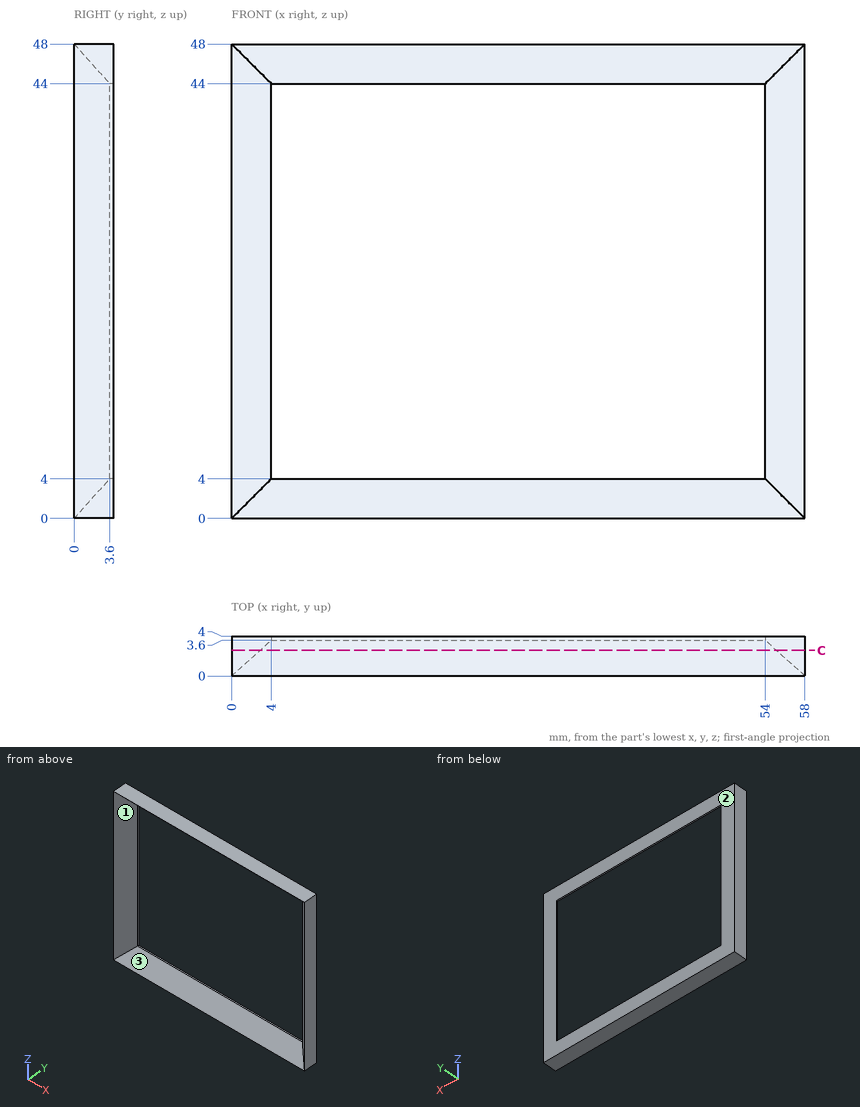
Source: three-view drawing plus pictorial views. Frame: mm from the lowest corner of the part. Coordinates: 2 decimals unless noted, no trailing zeros. Order: outer loops, then holes, each group sorted by start corner. A loop starts at its lowest first (then second) coordinate and runs counter-clockwise, first axis right, second up.
1) Section C-C (y = 2.6). Return loops of the section in (x, z).
Result sheet:
outline: (0, 0) - (58, 0) - (58, 48) - (0, 48) - close; hole (2.89, 2.89) - (55.11, 2.89) - (55.11, 45.11) - (2.89, 45.11) - close
2) Ray query, probe 1 along X at (y, z) = (0.65, 44.5); probe 2 along Z at (x, y) = (19, 2.8); probe 3 along X at (y, z) = (2.7, 17.5). Return the intervals inside material, ascending.
Result sheet:
probe 1: x = 0 to 0.72, 57.28 to 58
probe 2: z = 0 to 3.11, 44.89 to 48
probe 3: x = 0 to 3, 55 to 58
3) First-contact query: P1, Ø10, axis at x = 13, z = 34, coming from the -Y side. Flat tip, straight axial feed; report the tip coordinate or a pass-through.
Result sheet:
P1: passes through
4) Draft query along X for the marked faces 1, 2 and 3. Return one class per face: released by +X, released by -X, zero draft, split by the parting line, or undercut.
Result sheet:
face 1: undercut
face 2: zero draft
face 3: undercut
